Check sheet for the modelled part. Datum: model origin and axes. Units: mm. A direction names the side the tool comes from. Coordinates: 2 decimals unless noted, no trailing zeros. Loops run counter-clockwise (first coordinate to the right, second up) from the corner with the lowest first, then second, coordinate; pieces in that order, holes last. Notation, with made-up numbers: (38.25, 78) - (88.25, 78) arc R17 cw to (88.25, 97) - close; hole circle Ø3 at (-24.75, 60). An arc over 180 degrees is marked (long way). Use a Markdown table: item, result. Add a question column.
1) Sectioned sample at B-B, the plane x = 12. Enter the section's corners in (y, z).
2) Sectioned sample at A-A, the plane z = 0. Enter the section's corners in (x, y).
3) Sectioned sample at C-C, the plane y = -15. Enter the section's corners in (x, z), then the cut area to 3 significant figures.
4) Go/stop test with flat-tipped pins: P1, Ø2.5, axis at y = 5, z = 7.5, coming from the +X side; P2, Ø4, axis at x = 10, z = 5, coming from the -Y side; P3, Ø8, axis at y = -5.5, z = -8, coming from the +X side. Record where each tip stops, or that it passes through.
5) Draft check along Z on faces 1 (the flat face through (-4, 6, 12)), 2 (the flat face through (12.5, 1, -7)), 3 (the flat face through (-6, 8, 15)). Enter one of: pulls with the +Z half, pulls with the -Z half, needs draft (parallel to the pull), parting line crosses it, or undercut.
6) Tool access check on faces 4 (the flat face through (0, 11, -2)), 5 (the cylindrical face through (18.27, -16.28, 7.54)), 6 (the flat face through (12.5, -3, -7)). Record the directions out of +Z, -Z, +X, -X, +Y, -Y that give a thin tool (end or side, any length) a straight path to the whole face; none if there is none.
7) Thickness scan on line 1 (Z direction, x = 14.5, y = -8.5); line 2 (Y direction, x = -1.65, z = 0); line 3 (Y direction, x = 4, z = 4). Record the ranges inside material, lowest first.
8) Sectioned sample at D-D, the plane x = -6. Enter the section's corners in (y, z).
from build123d import *

# Parameters (mm, degrees)
SKETCH1_W                      = 20
SKETCH1_H                      = 15
BOSS_EXTRUDE1_DEPTH            = 15
SKETCH2_R                      = 2
BOSS_EXTRUDE2_DEPTH            = 5
BOSS_EXTRUDE3_DEPTH            = 15
BOSS_EXTRUDE3_DEPTH_BACK       = 12.5
FILLET1_R                      = 4
M3X0_5_TAPPED_HOLE1_D          = 2.5
M3X0_5_TAPPED_HOLE1_DEPTH      = 11
M3X0_5_TAPPED_HOLE1_TIP        = 0.751075774
CBORE_FOR_M3_SHCS1_D           = 3.4
CBORE_FOR_M3_SHCS1_DEPTH       = 9
CBORE_FOR_M3_SHCS1_CBORE_D     = 6.5
CBORE_FOR_M3_SHCS1_CBORE_DEPTH = 3
CBORE_FOR_M3_SHCS1_TIP         = 1.021463052
SKETCH8_R                      = 1.5
CUT_EXTRUDE1_DEPTH             = 2.5


with BuildPart() as part:
    # Sketch1 → Boss-Extrude1 (new body)
    with BuildSketch(Plane(origin=(0, 0, 0), x_dir=(0, 0, -1), z_dir=(1, 0, 0))):
        Rectangle(SKETCH1_W, SKETCH1_H)
    extrude(amount=BOSS_EXTRUDE1_DEPTH)

    # Sketch2 → Boss-Extrude2 (add)
    with BuildSketch(Plane.XY.offset(10)):
        with BuildLine():
            Line((15, -7.5), (10.015567122, -7.5))
            Line((10.015567122, -7.5), (10.015567122, -12.105755295))
            ThreePointArc((10.015567122, -12.105755295), (18.393285758, -16.172276101), (15, -7.5))
        make_face()
        with Locations((15, -12.5)):
            Circle(SKETCH2_R, mode=Mode.SUBTRACT)
    boss_extrude2 = extrude(amount=-BOSS_EXTRUDE2_DEPTH)

    # Mirror1: Boss-Extrude2 across plane
    add(boss_extrude2.mirror(Plane.XY))

    # Sketch3 → Boss-Extrude3 (add, two sides)
    with BuildSketch(Plane.XZ.offset(-7.5)) as boss_extrude3_sk:
        Polygon((-4, 10), (-4, 15), (-9, 15), (-9, -15), (-4, -15), (-4, -10), (0, -10), (0, 10), align=None)
    extrude(amount=BOSS_EXTRUDE3_DEPTH)
    extrude(boss_extrude3_sk.sketch, amount=-BOSS_EXTRUDE3_DEPTH_BACK)

    # Fillet1
    fillet1_edges = [part.edges().sort_by_distance(p)[0] for p in [
        (3.007783561, -7.5, 10),
        (3.007783561, -7.5, -10),
        (-6.5, -7.5, -15),
        (-6.5, -7.5, 15),
    ]]
    fillet(fillet1_edges, radius=FILLET1_R)

    # M3x0.5 Tapped Hole1
    with Locations(Plane(origin=(0, 0, 0), x_dir=(0, 0, -1), z_dir=(1, 0, 0))):
        with Locations((0, 13.90875121)):
            Hole(M3X0_5_TAPPED_HOLE1_D / 2, depth=M3X0_5_TAPPED_HOLE1_DEPTH)
            with Locations((0, 0, -(M3X0_5_TAPPED_HOLE1_DEPTH + M3X0_5_TAPPED_HOLE1_TIP / 2))):  # 118° drill point
                Cone(0, M3X0_5_TAPPED_HOLE1_D / 2, M3X0_5_TAPPED_HOLE1_TIP, mode=Mode.SUBTRACT)

    # CBORE for M3 SHCS1
    with Locations(Plane(origin=(0, 0, 0), x_dir=(0, 0, -1), z_dir=(1, 0, 0))):
        with Locations((0, 13.90875121)):
            CounterBoreHole(CBORE_FOR_M3_SHCS1_D / 2, CBORE_FOR_M3_SHCS1_CBORE_D / 2, CBORE_FOR_M3_SHCS1_CBORE_DEPTH, depth=CBORE_FOR_M3_SHCS1_DEPTH)
            with Locations((0, 0, -(CBORE_FOR_M3_SHCS1_DEPTH + CBORE_FOR_M3_SHCS1_TIP / 2))):  # 118° drill point
                Cone(0, CBORE_FOR_M3_SHCS1_D / 2, CBORE_FOR_M3_SHCS1_TIP, mode=Mode.SUBTRACT)

    # Sketch8 → Cut-Extrude1 (cut)
    with BuildSketch(Plane(origin=(15, 0, 0), x_dir=(0, 0, -1), z_dir=(1, 0, 0))):
        with Locations((-7.5, 5)):
            Circle(SKETCH8_R)
        with Locations((-2.5, 5)):
            Circle(SKETCH8_R)
        with Locations((2.5, 5)):
            Circle(SKETCH8_R)
        with Locations((7.5, 5)):
            Circle(SKETCH8_R)
        with Locations((-2.5, 1)):
            Circle(SKETCH8_R)
        with Locations((2.5, 1)):
            Circle(SKETCH8_R)
        with Locations((7.5, 1)):
            Circle(SKETCH8_R)
        with Locations((-2.5, -3)):
            Circle(SKETCH8_R)
        with Locations((2.5, -3)):
            Circle(SKETCH8_R)
        with Locations((7.5, -3)):
            Circle(SKETCH8_R)
        with Locations((-7.5, 1)):
            Circle(SKETCH8_R)
        with Locations((-7.5, -3)):
            Circle(SKETCH8_R)
    extrude(amount=-CUT_EXTRUDE1_DEPTH, mode=Mode.SUBTRACT)


solid = part.part
Solved:
| question | item | result |
|---|---|---|
| 1 | outline | (-16.5, -10) - (7.5, -10) - (7.5, 10) - (-16.5, 10) - (-16.5, 5) - (-7.5, 5) - (-7.5, -5) - (-16.5, -5) - close |
| 2 | outline | (-9, -7.5) - (15, -7.5) - (15, 7.5) - (0, 7.5) - (0, 10.66) - (-3, 10.66) - (-3, 12.21) - (-9, 12.21) - close; (-9, 15.61) - (-3, 15.61) - (-3, 17.16) - (0, 17.16) - (0, 20) - (-9, 20) - close |
| 3 | outline | (10.67, -10) - (19.33, -10) - (19.33, -5) - (10.67, -5) - close; (10.67, 5) - (19.33, 5) - (19.33, 10) - (10.67, 10) - close |
| 3 | area | 86.6 mm2 |
| 4 | P1 | stops at x = 12.5 |
| 4 | P2 | stops at y = -16.5 |
| 4 | P3 | stops at x = 19 |
| 5 | face 1 | needs draft |
| 5 | face 2 | undercut |
| 5 | face 3 | pulls with the +Z half |
| 6 | face 4 | +Z, -Z, +X, +Y |
| 6 | face 5 | +Z, -Z |
| 6 | face 6 | +X |
| 7 | line 1 | z = -10 to -5, 5 to 10 |
| 7 | line 2 | y = -7.5 to 10.66, 17.16 to 20 |
| 7 | line 3 | y = -7.5 to 7.5 |
| 8 | outline | (-7.5, -11) arc R4 ccw to (-3.5, -15) - (20, -15) - (20, 15) - (-3.5, 15) arc R4 ccw to (-7.5, 11) - close; hole circle Ø3.4 at (13.91, 0) |
